from build123d import *

# Parameters (mm, degrees)
F0_R     = 26.043361
F1_DEPTH = 76.2
F2_R     = 17.27391
F3_DEPTH = 152.4


with BuildPart() as f1:
    # F0 (on Front) → F1 (new body)
    with BuildSketch(Plane.XZ):
        with BuildLine():
            Line((-76.2, 0), (0, 0))
            Line((0, 0), (0, 50.8))
            Line((0, 50.8), (-149.225, 50.8))
            ThreePointArc((-149.225, 50.8), (-225.425, -25.4), (-149.225, -101.6))
            Line((-149.225, -101.6), (0, -101.6))
            Line((0, -101.6), (0, -50.8))
            Line((0, -50.8), (-76.2, -50.8))
            Line((-76.2, -50.8), (-76.2, 0))
        make_face()
        with Locations((-114.3, -25.472846)):
            Circle(F0_R, mode=Mode.SUBTRACT)
    extrude(amount=-F1_DEPTH)

    # F2 (on face) → F3 (cut)
    with BuildSketch(Plane.XY.offset(50.8)):
        with Locations((-52.560348, 37.856806)):
            Circle(F2_R)
    extrude(amount=-F3_DEPTH, mode=Mode.SUBTRACT)


solid = f1.part
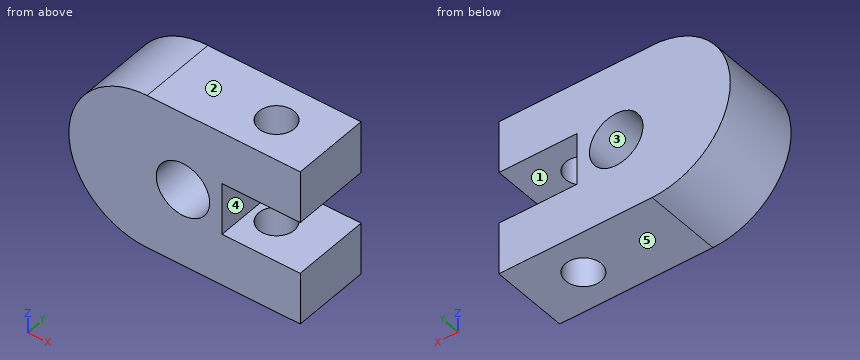
The model under review builds one solid part; all positions refer to its coordinate system, in mm. Face numbers are marked on the shaded views. A direction names the side the tool comes from. Give positions to 0.01 mm unless a question says otherwise; leave off trailing zeros. Order: outer loops, then holes, each group sorted by start corner. A loop starts at its lowest first (then second) coordinate and runs counter-clockwise, first axis right, second up. Notation, with made-up numbers: M 19.5,69 L 38.5,69 A14 cw 38.5,95 Z; hole C -23,38 d6. An arc over 180 degrees is marked long. Answer in a Markdown table with one row per item. Add a question column.
1. To check wall thickness, follow line 1 along Z through (x, y) = (-46, 60.5); line 2 along Z through (x, y) = (-114.3, 51.5); line 3 along X through (y, z) = (31, -86). State the ranges of each line that lie inside material, in increasing order.
2. Add section D-D on x = -63. State the section outline as (y, z) points.
3. Machinability: for the marked faces 1 and 2, which of the approach directions +Z, -Z, +X, -X, +Y, -Y give a long, thin tool a straight path to every point of the face, cutting with its end or side? Answer none if there is none.
4. Add section A-A on x = -114.3. State the section outline as (y, z) points, plus the area to 3 significant figures.
5. Add section B-B on z = -21. State the section outline as (x, y) points, plus the area to 3 significant figures.
6. Mouldability with a two-part tool opening along X and no side actions: class the marked faces 3, 4 and 5 as released by +X, released by -X, zero draft, split by the parting line, or undercut.
7. For pin 1 Ø6 at (y, z) = (59, 25.5) entering from -X; pin 2 Ø5 at (y, z) = (52.5, -26.5) entering from +X, all flat-tipped, find the tip position at first contact; note any pin that passes through.
8. Add section C-C on y = 63. State the section outline as (x, z) points (3 decimals).
The answers:
| question | item | result |
|---|---|---|
| 1 | line 1 | -101.6 to -50.8, 0 to 50.8 |
| 1 | line 2 | -101.6 to -51.52, 0.57 to 50.8 |
| 1 | line 3 | -195.42 to -68.42, -36.71 to 0 |
| 2 | outline | M 0,-101.6 L 24.09,-101.6 L 24.09,-50.8 L 0,-50.8 Z; M 0,0 L 24.09,0 L 24.09,50.8 L 0,50.8 Z; M 51.62,-101.6 L 76.2,-101.6 L 76.2,-50.8 L 51.62,-50.8 Z; M 51.62,0 L 76.2,0 L 76.2,50.8 L 51.62,50.8 Z |
| 3 | face 1 | +X, +Y, -Y |
| 3 | face 2 | +Z, +X, -X, +Y, -Y |
| 4 | outline | M 0,-101.6 L 76.2,-101.6 L 76.2,-51.52 L 0,-51.52 Z; M 0,0.57 L 76.2,0.57 L 76.2,50.8 L 0,50.8 Z |
| 4 | area | 7,640 mm2 |
| 5 | outline | M -225.3,0 L -139.96,0 L -139.96,76.2 L -225.3,76.2 Z; M -88.64,0 L -76.2,0 L -76.2,76.2 L -88.64,76.2 Z |
| 5 | area | 7,450 mm2 |
| 6 | face 3 | undercut |
| 6 | face 4 | released by +X |
| 6 | face 5 | zero draft |
| 7 | pin 1 | x = -208.49 |
| 7 | pin 2 | x = -76.2 |
| 8 | outline | M -149.225,-101.6 L 0,-101.6 L 0,-50.8 L -76.2,-50.8 L -76.2,0 L 0,0 L 0,50.8 L -149.225,50.8 A76.2 ccw Z; hole C -114.3,-25.473 d52.087 |
